Could you check a few things on this model? Use its own coordinates, in mm. Face numbers are marked on the shaded views. A direction names the side the tool comes from. Round coordinates to 2 decimals unless told otherwise and drop trailing zeros. Order: outer loops, then holes, each group sorted by start corner. A loop starts at its lowest first (then second) coordinate and runs counter-clockwise, first axis right, second up. Notation, with made-up numbers: (11.25, 69) - (38.25, 69) arc R16 cw to (38.25, 78) - close; hole circle Ø2 at (79, -15.5). An arc over 180 degrees is marked (long way). Use one line per item in the form item = value.
from build123d import *

# Parameters (mm, degrees)
F1_DEPTH  = 12.7
F3_DEPTH  = 12.7
F4_R      = 5.08
F5_R      = 3.9996078941
F6_DEPTH  = 25.4
F9_W      = 11.1263459548
F9_H      = 26.6221612692
F10_DEPTH = 12.7
F11_W     = 10.2434670553
F11_H     = 31.0408079531
F12_DEPTH = 12.7
F13_W     = 10.0882626139
F13_H     = 25.7638730109
F14_DEPTH = 12.7
F15_W     = 11.0194860026
F15_H     = 24.3218261437
F16_DEPTH = 12.7


with BuildPart() as f1:
    # F0 (on Front) → F1 (new body, symmetric)
    with BuildSketch(Plane.XZ):
        with BuildLine():
            ThreePointArc((-60.9433906042, 35.5109754222), (-56.1671910173, 39.4692096565), (-54.3759944375, 45.4081755227))
            ThreePointArc((-54.3759944375, 45.4081755227), (-57.5220599051, 53.0034494428), (-65.1173338252, 56.1495149105))
            ThreePointArc((-65.1173338252, 56.1495149105), (-75.6455235346, 43.2789518879), (-60.9433906042, 35.5109754222))
        make_face()
        with BuildLine():
            ThreePointArc((-58.3489453471, 45.4081755227), (-59.4776234248, 41.6658835524), (-62.4872270773, 39.1717004698))
            ThreePointArc((-62.4872270773, 39.1717004698), (-70.7570442257, 49.150467493), (-58.3489453471, 45.4081755227))
        make_face(mode=Mode.SUBTRACT)
        with BuildLine():
            ThreePointArc((-65.1173338252, 56.1495149105), (-57.5220599051, 53.0034494428), (-54.3759944375, 45.4081755227))
            ThreePointArc((-54.3759944375, 45.4081755227), (-56.1671910173, 39.4692096565), (-60.9433906042, 35.5109754222))
            Line((-60.9433906042, 35.5109754222), (-35.3970214505, -25.0642442118))
            ThreePointArc((-35.3970214505, -25.0642442118), (-24.9935148248, -26.0385154856), (-20.0531436301, -35.2458433869))
            Line((-20.0531436301, -35.2458433869), (20.1120705093, -35.2458433869))
            ThreePointArc((20.1120705093, -35.2458433869), (25.6970539708, -25.6418838342), (36.8063836854, -25.7461558165))
            Line((36.8063836854, -25.7461558165), (73.5966621145, 36.1738394268))
            ThreePointArc((73.5966621145, 36.1738394268), (68.7255805584, 48.2531038009), (79.0833194494, 56.1495149105))
            Line((79.0833194494, 56.1495149105), (-65.1173338252, 56.1495149105))
        make_face()
        with BuildLine():
            ThreePointArc((89.8246588372, 45.4081755227), (86.6785933696, 53.0034494428), (79.0833194494, 56.1495149105))
            ThreePointArc((79.0833194494, 56.1495149105), (68.7255805584, 48.2531038009), (73.5966621145, 36.1738394268))
            ThreePointArc((73.5966621145, 36.1738394268), (84.3956787796, 36.0724800376), (89.8246588372, 45.4081755227))
        make_face()
        with BuildLine():
            ThreePointArc((85.8517079276, 45.4081755227), (82.4307708597, 39.5255186699), (75.6260384765, 39.5893877739))
            ThreePointArc((75.6260384765, 39.5893877739), (75.7358680391, 51.2908323755), (85.8517079276, 45.4081755227))
        make_face(mode=Mode.SUBTRACT)
        with BuildLine():
            Line((-33.7332454412, -29.009368334), (-35.3970214505, -25.0642442118))
            ThreePointArc((-35.3970214505, -25.0642442118), (-37.2127625616, -44.4531712882), (-20.0531436301, -35.2458433869))
            Line((-20.0531436301, -35.2458433869), (-24.334750215, -35.2458433869))
            ThreePointArc((-24.334750215, -35.2458433869), (-34.8454306635, -40.8855537873), (-33.7332454412, -29.009368334))
        make_face()
        with BuildLine():
            ThreePointArc((-20.0531436301, -35.2458433869), (-24.9935148248, -26.0385154856), (-35.3970214505, -25.0642442118))
            Line((-35.3970214505, -25.0642442118), (-33.7332454412, -29.009368334))
            ThreePointArc((-33.7332454412, -29.009368334), (-27.3608467229, -29.6061329865), (-24.334750215, -35.2458433869))
            Line((-24.334750215, -35.2458433869), (-20.0531436301, -35.2458433869))
        make_face()
        with BuildLine():
            Line((34.6193465454, -29.4270556381), (36.8063836854, -25.7461558165))
            ThreePointArc((36.8063836854, -25.7461558165), (25.6970539708, -25.6418838342), (20.1120705093, -35.2458433869))
            Line((20.1120705093, -35.2458433869), (24.3936770943, -35.2458433869))
            ThreePointArc((24.3936770943, -35.2458433869), (27.8146141622, -29.3631865341), (34.6193465454, -29.4270556381))
        make_face()
        with BuildLine():
            ThreePointArc((42.2120606357, -35.2458433869), (40.7660251252, -29.7808317852), (36.8063836854, -25.7461558165))
            Line((36.8063836854, -25.7461558165), (34.6193465454, -29.4270556381))
            ThreePointArc((34.6193465454, -29.4270556381), (37.0447224253, -31.8983919766), (37.9304540507, -35.2458433869))
            ThreePointArc((37.9304540507, -35.2458433869), (31.1620655725, -42.0142318651), (24.3936770943, -35.2458433869))
            Line((24.3936770943, -35.2458433869), (20.1120705093, -35.2458433869))
            ThreePointArc((20.1120705093, -35.2458433869), (31.1620655725, -46.2958384501), (42.2120606357, -35.2458433869))
        make_face()
    extrude(amount=F1_DEPTH, both=True)

    # F2 (on face) → F3 (cut)
    with BuildSketch(Plane.XZ.offset(12.7)):
        Polygon((-41.8454812837, 56.1495149105), (-18.0603434561, -0.2494958163), (23.4314955848, -0.2494958163), (56.9414353, 56.1495149105), align=None)
    extrude(amount=-F3_DEPTH, mode=Mode.SUBTRACT)

    # F4
    f4_edges = [f1.edges().sort_by_distance(p)[0] for p in [
        (23.431496, -6.35, -0.249496),
        (-18.060343, -6.35, -0.249496),
    ]]
    fillet(f4_edges, radius=F4_R)

    # F5 (on face) → F6 (cut)
    with BuildSketch(Plane.XZ):
        with Locations((-12.5058135018, 12.8743648529)):
            Circle(F5_R)
        with Locations((12.5058135018, 12.8743648529)):
            Circle(F5_R)
    extrude(amount=-F6_DEPTH, mode=Mode.SUBTRACT)

    # F9 (on face) → F10 (cut, symmetric)
    with BuildSketch(Plane(origin=(38.5090528963, 0, -22.8804729802), x_dir=(0, 1, 0), z_dir=(0.8597006167, 0, -0.5107982475))):
        with Locations((-0.0419579446, 78.6430984735)):
            Rectangle(F9_W, F9_H)
    extrude(amount=F10_DEPTH, both=True, mode=Mode.SUBTRACT)

    # F11 (on face) → F12 (cut, symmetric)
    with BuildSketch(Plane(origin=(38.5090528963, 0, -22.8804729802), x_dir=(0, 1, 0), z_dir=(0.8597006167, 0, -0.5107982475))):
        with Locations((0.6208214909, -17.5293247448)):
            Rectangle(F11_W, F11_H)
    extrude(amount=F12_DEPTH, both=True, mode=Mode.SUBTRACT)

    # F13 (on face) → F14 (cut, symmetric)
    with BuildSketch(Plane(origin=(-39.0262986274, 0, -16.4585491801), x_dir=(0, -1, 0), z_dir=(-0.9214121017, 0, -0.3885868485))):
        with Locations((0.0776012894, 66.4450954646)):
            Rectangle(F13_W, F13_H)
    extrude(amount=F14_DEPTH, both=True, mode=Mode.SUBTRACT)

    # F15 (on face) → F16 (cut, symmetric)
    with BuildSketch(Plane(origin=(-39.0262986274, 0, -16.4585491801), x_dir=(0, -1, 0), z_dir=(-0.9214121017, 0, -0.3885868485))):
        with Locations((-0.2328096889, -21.5005939982)):
            Rectangle(F15_W, F15_H)
    extrude(amount=F16_DEPTH, both=True, mode=Mode.SUBTRACT)


solid = f1.part
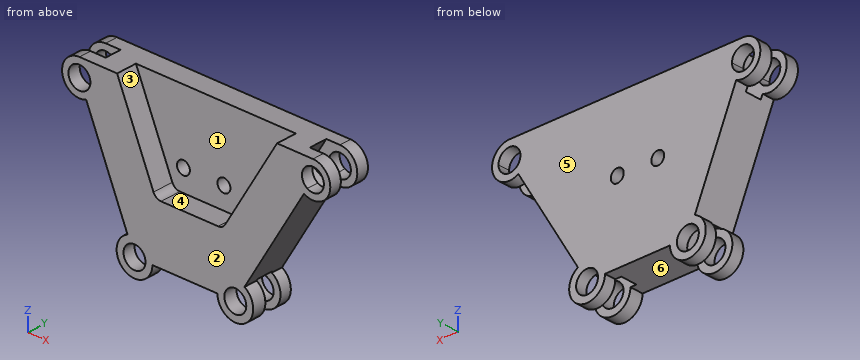
Item 1: Imagine slicing it at A-A on z = -38.5. State how many separate pieces and enclosed holes the cut face has, plus the area to 3 significant figures.
Found:
separate_pieces = 8
enclosed_holes = 0
area = 273 mm2
Item 2: If we mould it in two halves opening along X, with no side actions, what happens to the marked faces 1, 2 and 3? For each: released by +X, released by -X, zero draft, split by the parting line, or undercut.
Found:
face_1 = undercut
face_2 = zero draft
face_3 = undercut
Item 3: I need wall thicknesses on L1, parallel to X at y = 8.25, z = 40.5; L2, parallel to X at y = -6, z = 36; L3, parallel to X at y = -8, z = 45.5. Which ranges of each line are inside material? Lowest first, please.
Found:
L1 = -74.67 to -69.78, -60.46 to 74.42, 83.74 to 88.64
L2 = -70.3 to -33.35, 44.97 to 73.49, 73.9 to 84.27
L3 = -75.86 to -71.89, -58.35 to -37.35, 50.61 to 72.32, 85.85 to 89.82
Item 4: Will these pins go through, and if not, where does the flat tip stop? P1, Ø1.5, axis at x = 1, y = -6.5, coming from the +Z side; P2, Ø5, axis at x = -51, y = -2, coming from the -Z side; P3, Ø5, axis at x = 34, y = 4, coming from the -Z side.
Found:
P1 = -0.25
P2 = 6.01
P3 = -46.25
Item 5: Imagine slicing it at D-D on x = -13. Please give me the cut outline in (y, z).
Found:
outline = (-12.7, -35.25) - (12.7, -35.25) - (12.7, 8.91) - (0, 8.91) - (0, -0.25) - (-12.7, -0.25) - close; (0, 16.84) - (12.7, 16.84) - (12.7, 56.15) - (0, 56.15) - close
Item 6: For the marked faces 4, 5 and 6, which set-ups out of +Z, -Z, +X, -X, +Y, -Y let a thin tool reach every point of the face, with its end or its side?
Found:
face_4 = +Z, -Y
face_5 = +Z, -Z, +X, -X, +Y
face_6 = -Z, +Y, -Y
Item 7: Imagine slicing it at B-B on y = -2.25. Please give me the cut outline in (x, z).
Found:
outline = (-59.84, 32.9) - (-35.4, -25.06) - (-23.7, -20.13) - (-17.32, -35.25) - (16.39, -35.25) - (26.56, -18.12) - (37.48, -24.61) - (71.88, 33.29) - (60.96, 39.77) - (70.69, 56.15) - (56.94, 56.15) - (24.91, 2.24) arc R5.08 cw to (20.54, -0.25) - (-14.69, -0.25) arc R5.08 cw to (-19.37, 2.86) - (-41.85, 56.15) - (-55.86, 56.15) - (-48.14, 37.83) - close
Item 8: Imagine slicing it at C-C on x = 33. Please give me the cut outline in (y, z).
Found:
outline = (-12.7, -46.14) - (-4.5, -46.14) - (-4.5, -41.76) - (-12.7, -41.76) - close; (-12.7, -28.73) - (-4.5, -28.73) - (-4.5, -21.94) - (5.74, -21.94) - (5.74, -28.73) - (12.7, -28.73) - (12.7, 56.15) - (0, 56.15) - (0, 15.85) - (-12.7, 15.85) - close; (5.74, -46.14) - (12.7, -46.14) - (12.7, -41.76) - (5.74, -41.76) - close
